Could you check a few things on this model? Use its own coordinates, in mm. A direction names the side the tool comes from. Round coordinates to 2 decimals unless told otherwise and drop trailing zeros. Write each loop counter-clockwise with the first axis right and the second up, starting at its lowest first coordinate (ties: lowest second). Pieces come first, ordered by that corner, then holes. Notation, with made-up numbers: (-3.75, -13) -> (44.25, -13) arc R17 cw to (44.25, 0) -> close; hole circle Ø2 at (56, -0.75). An arc over 180 degrees is marked (long way). Answer in a Markdown table with one row per item. Add a question column.
```python
from build123d import *

# Parameters (mm, degrees)
BOSS_EXTRUDE1_DEPTH = 10
CUT_EXTRUDE3_DEPTH  = 5
SKETCH5_W           = 10
SKETCH5_H           = 49.5
BOSS_EXTRUDE2_DEPTH = 5
FILLET1_R           = 10
SKETCH6_W           = 10
SKETCH6_H           = 300
CUT_EXTRUDE5_DEPTH  = 4
SKETCH8_W           = 10
SKETCH8_H           = 30
BOSS_EXTRUDE3_DEPTH = 4
SKETCH10_W          = 10
SKETCH10_H          = 300
CUT_EXTRUDE6_DEPTH  = 4
SKETCH11_W          = 10
SKETCH11_H          = 30
BOSS_EXTRUDE4_DEPTH = 4


with BuildPart() as part:
    # Sketch1 → Boss-Extrude1 (new body)
    with BuildSketch(Plane.XY):
        with BuildLine():
            Line((0, 0), (250, 0))
            Line((250, 0), (285.355339059, 35.355339059))
            Line((285.355339059, 35.355339059), (285.355339059, 326.955339059))
            ThreePointArc((285.355339059, 326.955339059), (243.560486982, 353.188356712), (195, 361.955339059))
            Line((195, 361.955339059), (55, 361.955339059))
            ThreePointArc((55, 361.955339059), (6.439513018, 353.188356712), (-35.355339059, 326.955339059))
            Line((-35.355339059, 326.955339059), (-35.355339059, 35.355339059))
            Line((-35.355339059, 35.355339059), (0, 0))
        make_face()
    extrude(amount=BOSS_EXTRUDE1_DEPTH)

    # Sketch4 → Cut-Extrude3 (cut)
    with BuildSketch(Plane.XY.offset(10)):
        with BuildLine():
            Line((-25.355339059, 39.497474683), (4.142135624, 10))
            Line((4.142135624, 10), (245.857864376, 10))
            Line((245.857864376, 10), (275.355339059, 39.497474683))
            Line((275.355339059, 39.497474683), (275.355339059, 322.508901748))
            ThreePointArc((275.355339059, 322.508901748), (237.921386907, 344.627720124), (195.062911656, 351.955339059))
            Line((195.062911656, 351.955339059), (54.937088344, 351.955339059))
            ThreePointArc((54.937088344, 351.955339059), (12.078613093, 344.627720124), (-25.355339059, 322.508901748))
            Line((-25.355339059, 322.508901748), (-25.355339059, 39.497474683))
        make_face()
    extrude(amount=-CUT_EXTRUDE3_DEPTH, mode=Mode.SUBTRACT)

    # Sketch5 → Boss-Extrude2 (add)
    with BuildSketch(Plane.XY.offset(5)):
        with Locations((59.644660941, 164.705339059)):
            Rectangle(SKETCH5_W, SKETCH5_H)
        with Locations((190.355339059, 164.705339059)):
            Rectangle(SKETCH5_W, SKETCH5_H)
    extrude(amount=BOSS_EXTRUDE2_DEPTH)

    # Fillet1
    fillet1_edges = [part.edges().sort_by_distance(p)[0] for p in [
        (-35.355339059, 35.355339059, 5),
        (-35.355339059, 326.955339059, 5),
        (285.355339059, 326.955339059, 5),
        (285.355339059, 35.355339059, 5),
        (250, 0, 5),
        (0, 0, 5),
    ]]
    fillet(fillet1_edges, radius=FILLET1_R)

    # Sketch6 → Cut-Extrude5 (cut)
    with BuildSketch(Plane(origin=(0, 0, 0), x_dir=(-1, 0, 0), z_dir=(0, 0, -1))):
        with Locations((-230.355339059, 180)):
            Rectangle(SKETCH6_W, SKETCH6_H)
    extrude(amount=-CUT_EXTRUDE5_DEPTH, mode=Mode.SUBTRACT)

    # Sketch8 → Boss-Extrude3 (add)
    with BuildSketch(Plane(origin=(0, 0, 4), x_dir=(-1, 0, 0), z_dir=(0, 0, -1))):
        with Locations((-230.355339059, 285)):
            Rectangle(SKETCH8_W, SKETCH8_H)
        with Locations((-230.355339059, 75)):
            Rectangle(SKETCH8_W, SKETCH8_H)
    extrude(amount=BOSS_EXTRUDE3_DEPTH)

    # Sketch10 → Cut-Extrude6 (cut)
    with BuildSketch(Plane(origin=(0, 0, 0), x_dir=(-1, 0, 0), z_dir=(0, 0, -1))):
        with Locations((-19.644660941, 180)):
            Rectangle(SKETCH10_W, SKETCH10_H)
    extrude(amount=-CUT_EXTRUDE6_DEPTH, mode=Mode.SUBTRACT)

    # Sketch11 → Boss-Extrude4 (add)
    with BuildSketch(Plane(origin=(0, 0, 4), x_dir=(-1, 0, 0), z_dir=(0, 0, -1))):
        with Locations((-19.644660941, 75)):
            Rectangle(SKETCH11_W, SKETCH11_H)
        with Locations((-19.644660941, 285)):
            Rectangle(SKETCH11_W, SKETCH11_H)
    extrude(amount=BOSS_EXTRUDE4_DEPTH)


solid = part.part
```
(1) Suppose I cut it at C-C, the plane z = 2. State how many separate pieces and enclosed holes the cut face has, then the cut area to 3 significant figures.
(2) I need wall thicknesses on L1, parallel to X at y = 268.5, z = 2.75; L2, parallel to X at y = 153, z = 7.25; L3, parallel to X at y = 200.5, z = 6. Which ranges of each line are inside material? Lowest first, please.
(3) Suppose I cut it at A-A, the plane y = 54.5. Please give me the cut outline in (x, z).
(4) If we mould it in two halves opening along Y, with no side actions, what happens to faces 4 (the face through (230, 45, 4)), 5 (the face through (126, 361.955, 5)), 6 (the face through (190, 165, 10))? For each: pulls with the +Y half, pulls with the -Y half, needs draft (parallel to the pull), parting line crosses it, or undercut.
(5) Suppose I cut it at D-D, the plane x = 34.5. Please give me the cut outline in (y, z).
(6) On a 3-axis mill with a long thin cutter (end or side, diameter ignored), from which of +Z, -Z, +X, -X, +Y, -Y can I reach the whole of each face in a straight line? I mean faces 1 (the face through (20, 45, 4)), 2 (the face through (285.355, 179, 5)), 3 (the face through (238.496, 344.415, 7.535)). Say none if no direction works.
(7) For P1, Ø3, axis at x = 18.5, y = 320.5, coming from the -Z side; P2, Ø3, axis at x = 20.5, z = 3, coming from the +Y side; P3, Ø1, axis at y = 38.5, z = 3.5, coming from the -X side, each with a flat end and sliding along its axis, tell me the tip position at first contact or that it passes through.
(8) Suppose I cut it at B-B, the plane x = 171. Please give me the cut outline in (y, z), then the cut area to 3 significant figures.
Response:
| question | item | result |
|---|---|---|
| 1 | separate pieces | 1 |
| 1 | enclosed holes | 6 |
| 1 | area | 108,000 mm² |
| 2 | L1 | -35.36 to 14.64, 24.64 to 225.36, 235.36 to 285.36 |
| 2 | L2 | -35.36 to -25.36, 54.64 to 64.64, 185.36 to 195.36, 275.36 to 285.36 |
| 2 | L3 | -35.36 to -25.36, 275.36 to 285.36 |
| 3 | outline | (-35.36, 0) -> (14.64, 0) -> (14.64, 4) -> (24.64, 4) -> (24.64, 0) -> (225.36, 0) -> (225.36, 4) -> (235.36, 4) -> (235.36, 0) -> (285.36, 0) -> (285.36, 10) -> (275.36, 10) -> (275.36, 5) -> (-25.36, 5) -> (-25.36, 10) -> (-35.36, 10) -> close |
| 4 | face 4 | undercut |
| 4 | face 5 | pulls with the +Y half |
| 4 | face 6 | needs draft |
| 5 | outline | (0, 0) -> (360.58, 0) -> (360.58, 10) -> (350.47, 10) -> (350.47, 5) -> (10, 5) -> (10, 10) -> (0, 10) -> close |
| 6 | face 1 | -Z |
| 6 | face 2 | +Z, -Z, +X, +Y, -Y |
| 6 | face 3 | +Z |
| 7 | P1 | z = 4 |
| 7 | P2 | y = 358.12 |
| 7 | P3 | x = -35.34 |
| 8 | outline | (0, 0) -> (361.96, 0) -> (361.96, 10) -> (351.96, 10) -> (351.96, 5) -> (10, 5) -> (10, 10) -> (0, 10) -> close |
| 8 | area | 1,910 mm² |
